Model file for the job. Use its own axes, mm. A direction names the side the tool comes from. Round coordinates to 2 decimals unless told otherwise and drop trailing zeros. Order: outer loops, then holes, each group sorted by start corner. A loop starts at its lowest first (then second) coordinate and runs counter-clockwise, first axis right, second up. Notation, with made-up numbers: (-25, -35.75) - (22, -35.75) arc R20 ccw to (22, -8.75) - close; hole circle Ø9 at (-0.5, 33.5). An arc over 180 degrees is marked (long way). Use one line per item in the form item = value.
from build123d import *

# Parameters (mm, degrees)
F1_DEPTH = 6.35
F2_R     = 15.8115
F2_R_2   = 14.351
F3_DEPTH = 6.35


with BuildPart() as f1:
    # F0 (on Top) → F1 (new body)
    with BuildSketch(Plane.XY):
        Polygon((0.360184, -41.58426), (36.193117, -20.480202), (35.832934, 21.104058), (-0.360184, 41.58426), (-36.193117, 20.480202), (-35.832934, -21.104058), align=None)
    extrude(amount=F1_DEPTH)

    # F2 (on face) → F3 (join)
    with BuildSketch(Plane.XY.offset(6.35)):
        Circle(F2_R)
        Circle(F2_R_2, mode=Mode.SUBTRACT)
    extrude(amount=F3_DEPTH)


solid = f1.part
(1) Pull direction Y, two halves, no side cores. Call faces 1 (the face through (0, 0, 6.35)), 2 (the face through (-4, -14, 12.7)), 3 (the face through (17.99, 31.2, 3.13)): released by +Y, released by -Y, zero draft, split by the parting line, or undercut.
Report:
face_1 = undercut
face_2 = zero draft
face_3 = released by +Y
(2) Pin check, flat tips, straight feed: pin 1 (1.5 mm diameter, centred on x = 28, y = 1, fed in from -Z); pin 2 (5 mm diameter, centred on x = 14.5, z = 2.5, fed in from +Y); pin 3 (5 mm diameter, centred on x = -5, z = 9.5, fed in from +Y); pin 4 (8 mm diameter, centred on x = 21.5, y = -26.5, fed in from +Z). Stop position of each tip, or through.
Report:
pin_1 = 0
pin_2 = 34.59
pin_3 = 15.61
pin_4 = 6.35
(3) Slice it at B-B on x = 6. Give the cut face in (y, z).
Report:
outline = (-38.26, 0) - (37.99, 0) - (37.99, 6.35) - (14.63, 6.35) - (14.63, 12.7) - (13.04, 12.7) - (13.04, 6.35) - (-13.04, 6.35) - (-13.04, 12.7) - (-14.63, 12.7) - (-14.63, 6.35) - (-38.26, 6.35) - close
(4) Probe probe 1 along Y at (x, z) = (0, 8.75); probe 2 along Z at (x, y) = (10, 34.5); probe 3 along Y at (x, z) = (-5, 7). List the from-to ranges inside material, lowest first. Write a range as [from, to].
Report:
probe_1 = [-15.81, -14.35], [14.35, 15.81]
probe_2 = [0, 6.35]
probe_3 = [-15, -13.45], [13.45, 15]
(5) Slice it at A-A on z = 10.5. Give the cut face in (x, y), then the cut area to 3 significant figures.
Report:
outline = circle Ø31.62 at (0, 0); hole circle Ø28.7 at (0, 0)
area = 138 mm2
(6) Tool access for faces 4 (the face through (-3.11, -14.01, 9.48)), 5 (the face through (-1, 1, 0)): list every direction of +Z, -Z, +X, -X, +Y, -Y with a clear straight run to the whole face (end or side of a thin tool).
Report:
face_4 = +Z
face_5 = -Z, +X, -X, +Y, -Y
(7) Slice it at C-C on y = 0. Give the cut face in (x, z), then the cut area to 3 significant figures.
Report:
outline = (-36.02, 0) - (36.02, 0) - (36.02, 6.35) - (15.81, 6.35) - (15.81, 12.7) - (14.35, 12.7) - (14.35, 6.35) - (-14.35, 6.35) - (-14.35, 12.7) - (-15.81, 12.7) - (-15.81, 6.35) - (-36.02, 6.35) - close
area = 476 mm2
(8) Slice it at D-D on x = -21. Give the cut face in (y, z), then the cut area to 3 significant figures.
Report:
outline = (-29.5, 0) - (29.43, 0) - (29.43, 6.35) - (-29.5, 6.35) - close
area = 374 mm2
